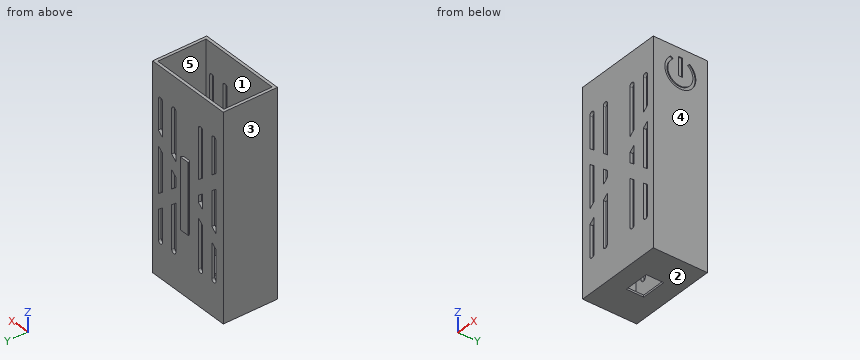
from build123d import *

# Parameters (mm, degrees)
F0_W      = 92
F0_H      = 56
F0_W_2    = 86
F0_H_2    = 50
F1_DEPTH  = 210
F2_W      = 86
F2_H      = 50
F3_DEPTH  = 2
F4_W      = 26
F4_H      = 18
F5_DEPTH  = 25
F7_START  = -65.3
F7_DEPTH  = 72.4
F8_SIZE   = 1
F10_DEPTH = 56.001
F12_DEPTH = 3
F13_START = -53
F13_DEPTH = 3
F14_W     = 4
F14_H     = 19.115075469
F15_DEPTH = 1


with BuildPart() as f1:
    # F0 (on Top) → F1 (new body)
    with BuildSketch(Plane.XY):
        with Locations((7.8588197877, 5.9614046181)):
            Rectangle(F0_W, F0_H)
        with Locations((7.8588197877, 5.9614046181)):
            Rectangle(F0_W_2, F0_H_2, mode=Mode.SUBTRACT)
    extrude(amount=F1_DEPTH)

    # F2 (on Top) → F3 (join)
    with BuildSketch(Plane.XY):
        with Locations((7.8588197877, 5.9614046181)):
            Rectangle(F2_W, F2_H)
    extrude(amount=F3_DEPTH)

    # F4 (on face) → F5 (cut)
    with BuildSketch(Plane.XY.offset(2)):
        with Locations((7.8588197877, 5.9614046181)):
            Rectangle(F4_W, F4_H)
    extrude(amount=-F5_DEPTH, mode=Mode.SUBTRACT)

    # F6 (on face) → F7 (join)
    with BuildSketch(Plane(origin=(0, 0, 0), x_dir=(1, 0, 0), z_dir=(0, 0, -1)).offset(F7_START)):
        Polygon((12.8588197877, -33.9614046181), (5.8588197877, -33.9614046181), (3.3588197877, -36.4614046181), (15.3588197877, -36.4614046181), align=None)
    extrude(amount=-F7_DEPTH)

    # F8
    f8_edges = [f1.edges().sort_by_distance(p)[0] for p in [
        (15.35882, 36.461405, 101.5),
        (3.35882, 36.461405, 101.5),
    ]]
    chamfer(f8_edges, length=F8_SIZE)

    # F9 (on face) → F10 (cut, through all)
    with BuildSketch(Plane(origin=(0, 33.9614046181, 0), x_dir=(-1, 0, 0), z_dir=(0, 1, 0))):
        with BuildLine():
            Line((-23.6102305163, 36.7792584002), (-23.6102305163, 176.6065955162))
            ThreePointArc((-23.6102305163, 176.6065955162), (-26.284525152, 179.2808901519), (-28.9588197877, 176.6065955162))
            Line((-28.9588197877, 176.6065955162), (-28.9588197877, 36.7792584002))
            ThreePointArc((-28.9588197877, 36.7792584002), (-26.284525152, 34.1049637645), (-23.6102305163, 36.7792584002))
        make_face()
        with BuildLine():
            Line((11.1897694837, 36.7792584002), (11.1897694837, 176.6065955162))
            ThreePointArc((11.1897694837, 176.6065955162), (8.515474848, 179.2808901519), (5.8411802123, 176.6065955162))
            Line((5.8411802123, 176.6065955162), (5.8411802123, 36.7792584002))
            ThreePointArc((5.8411802123, 36.7792584002), (8.515474848, 34.1049637645), (11.1897694837, 36.7792584002))
        make_face()
        with BuildLine():
            Line((28.5897694837, 36.7792584002), (28.5897694837, 176.6065955162))
            ThreePointArc((28.5897694837, 176.6065955162), (25.915474848, 179.2808901519), (23.2411802123, 176.6065955162))
            Line((23.2411802123, 176.6065955162), (23.2411802123, 36.7792584002))
            ThreePointArc((23.2411802123, 36.7792584002), (25.915474848, 34.1049637645), (28.5897694837, 36.7792584002))
        make_face()
        with BuildLine():
            ThreePointArc((-41.0102305163, 176.6065955162), (-43.684525152, 179.2808901519), (-46.3588197877, 176.6065955162))
            Line((-46.3588197877, 176.6065955162), (-46.3588197877, 36.7792584002))
            ThreePointArc((-46.3588197877, 36.7792584002), (-43.684525152, 34.1049637645), (-41.0102305163, 36.7792584002))
            Line((-41.0102305163, 36.7792584002), (-41.0102305163, 176.6065955162))
        make_face()
    extrude(amount=-F10_DEPTH, mode=Mode.SUBTRACT)

    # F11 (on face) → F12 (join)
    with BuildSketch(Plane.XZ.offset(22.0385953819)):
        Polygon((-38.1411802123, 151.7051618288), (-38.1411802123, 136.1901685596), (-1.6069489009, 106.2492112246), (7.8588197877, 114.0067078593), align=None)
        Polygon((7.8588197877, 114.0067078593), (-1.6069489009, 106.2492112246), (7.8588197877, 98.49171459), (17.3245884762, 106.2492112246), align=None)
        Polygon((7.8588197877, 98.49171459), (-1.6069489009, 106.2492112246), (-38.1411802123, 76.3082538897), (-38.1411802123, 60.7932606204), align=None)
        Polygon((17.3245884762, 106.2492112246), (7.8588197877, 98.49171459), (53.8588197877, 60.7932606204), (53.8588197877, 76.3082538897), align=None)
        Polygon((53.8588197877, 151.7051618288), (7.8588197877, 114.0067078593), (17.3245884762, 106.2492112246), (53.8588197877, 136.1901685596), align=None)
    extrude(amount=-F12_DEPTH)

    # F11 (on face) → F13 (join)
    with BuildSketch(Plane.XZ.offset(22.0385953819).offset(F13_START)):
        Polygon((-38.1411802123, 151.7051618288), (-38.1411802123, 136.1901685596), (-1.6069489009, 106.2492112246), (7.8588197877, 114.0067078593), align=None)
        Polygon((7.8588197877, 114.0067078593), (-1.6069489009, 106.2492112246), (7.8588197877, 98.49171459), (17.3245884762, 106.2492112246), align=None)
        Polygon((7.8588197877, 98.49171459), (-1.6069489009, 106.2492112246), (-38.1411802123, 76.3082538897), (-38.1411802123, 60.7932606204), align=None)
        Polygon((17.3245884762, 106.2492112246), (7.8588197877, 98.49171459), (53.8588197877, 60.7932606204), (53.8588197877, 76.3082538897), align=None)
        Polygon((53.8588197877, 151.7051618288), (7.8588197877, 114.0067078593), (17.3245884762, 106.2492112246), (53.8588197877, 136.1901685596), align=None)
    extrude(amount=-F13_DEPTH)

    # F14 (on face) → F15 (cut)
    with BuildSketch(Plane.YZ.offset(53.8588197877)):
        with BuildLine():
            Line((-1.4880481935, 196.3340106044), (-3.7893929464, 198.3656088747))
            ThreePointArc((-3.7893929464, 198.3656088747), (5.9614046181, 169.6801074319), (15.7122021826, 198.3656088747))
            Line((15.7122021826, 198.3656088747), (13.4108574297, 196.3340106044))
            ThreePointArc((13.4108574297, 196.3340106044), (5.9614046181, 172.6801074319), (-1.4880481935, 196.3340106044))
        make_face()
        with Locations((6.0325704031, 191.79122895)):
            Rectangle(F14_W, F14_H)
    extrude(amount=-F15_DEPTH, mode=Mode.SUBTRACT)


solid = f1.part
The model under review builds one solid part; all positions refer to its coordinate system, in mm. Face numbers are marked on the shaded views. A direction names the side the tool comes from. Coordinates: 2 decimals unless noted, no trailing zeros. Write each loop counter-clockwise with the first axis right and the second up, starting at its lowest first coordinate (ties: lowest second). Pieces come first, ordered by that corner, then holes. Notation, with made-up numbers: (-7, -27.75) - (33, -27.75) arc R27 cw to (33, -9.75) - close; hole circle Ø8 at (-7.5, 25.25). An arc over 180 degrees is marked (long way). Answer as a JSON object with one key per item and string values. Group by question number.
1. Add section D-D (x = -18). Give the boundary of the cut face in (y, z).
2. Add section C-C (x = 0). Give the boundary of the cut face in (y, z), plus the area to 3 significant figures.
3. Clearance check with flat-ended pins moving along their axes: pin 1 Ø2 at (x, y) = (11.5, 34.5) entering from +Z; pin 2 Ø2 at (x, z) = (14, 1) entering from +Y; pin 3 Ø2 at (x, y) = (11, -7.5) entering from +Z; pin 4 Ø3 at (y, z) = (6.5, 196) entering from +X. State where each tip first meets the part, or that it passes through.
4. Add section A-A (z = 24). Give the boundary of the cut face in (x, y).
5. Add section B-B (y = 2). Give the boundary of the cut face in (x, z), plus the area to 3 significant figures.
6. Machinability: for the marked faces 4 and 5, which of the approach directions +Z, -Z, +X, -X, +Y, -Y give a long, thin tool a straight path to every point of the face, cutting with its end or side? Answer none if there is none.
7. Mouldability with a two-part tool opening along X and no side actions: class the marked faces 1, 2 and 3 as pulls with the +X half, pulls with the -X half, needs draft (parallel to the pull), parting line crosses it, or undercut.
8. To check wall thickness, follow probe 1 along X at (y, z) = (3.5, 94); probe 2 along Y at (x, z) = (39, 201); probe 3 along Y at (x, z) = (6, 67). State the ranges of each line that lie inside material, in increasing order.
Findings:
{
 "1": {"outline": "(-22.04, 0) - (33.96, 0) - (33.96, 210) - (30.96, 210) - (30.96, 2) - (-19.04, 2) - (-19.04, 210) - (-22.04, 210) - close"},
 "2": {"outline": "(-22.04, 0) - (-3.04, 0) - (-3.04, 2) - (-19.04, 2) - (-19.04, 210) - (-22.04, 210) - close; (14.96, 0) - (33.96, 0) - (33.96, 210) - (30.96, 210) - (30.96, 2) - (14.96, 2) - close", "area": "1,320 mm²"},
 "3": {"pin 1": "z = 210", "pin 2": "y = 33.96", "pin 3": "z = 2", "pin 4": "x = 52.86"},
 "4": {"outline": "(-38.14, -22.04) - (53.86, -22.04) - (53.86, 33.96) - (-38.14, 33.96) - close; hole (-35.14, -19.04) - (50.86, -19.04) - (50.86, 30.96) - (-35.14, 30.96) - close"},
 "5": {"outline": "(-38.14, 0) - (-5.14, 0) - (-5.14, 2) - (-35.14, 2) - (-35.14, 210) - (-38.14, 210) - close; (20.86, 0) - (53.86, 0) - (53.86, 170.18) - (52.86, 170.18) - (52.86, 173.3) - (53.86, 173.3) - (53.86, 210) - (50.86, 210) - (50.86, 2) - (20.86, 2) - close", "area": "1,380 mm²"},
 "6": {"face 4": "+Z, -Z, +X, +Y, -Y", "face 5": "+Z"},
 "7": {"face 1": "undercut", "face 2": "needs draft", "face 3": "pulls with the -X half"},
 "8": {"probe 1": "-38.14 to -35.14, 50.86 to 53.86", "probe 2": "-22.04 to -19.04, 30.96 to 33.96", "probe 3": "-22.04 to -19.04, 30.96 to 36.46"}
}
